Here's how the part is built. I have some questions about the finished solid (model axes, mm). A direction names the side the tool comes from. Coordinates: 2 decimals unless noted, no trailing zeros. Loops run counter-clockwise (first coordinate to the right, second up) from the corner with the lowest first, then second, coordinate; pieces in that order, holes last. Notation, with made-up numbers: M -2.5,-1 L 31.5,-1 A17 cw 31.5,19 Z; hole C 32,33.25 d5. An arc over 180 degrees is marked long. Use CSV: the item, a comma, the result in double quotes. Start each with the question number.
Q1. For pin 1 Ø15 at (x, z) = (669, -549.5) entering from +Y; pin 2 Ø15 at (y, z) = (270.5, -512) entering from -X; pin 3 Ø15 at (x, z) = (668.5, -291) entering from -Y; pin 4 Ø4 at (x, y) = (178, 278.5) entering from +Z, each with a flat end and sliding along its axis, tell me the tip position at first contact or that it passes through.
Q2. If we section it at C-C (x = 64.5): Please give me the cut outline in (y, z), and give its area (3 significant figures).
Q3. If we mould it in two halves opening along X, with no side actions, what happens to faces 1 (the flat face through (-698.5, -267, -389)), 2 (the flat face through (-673, 292.1, -389)), 3 (the flat face through (647.7, 266, -389))? For each: +X half, -X half, draft (parallel to the pull), parting line (faces both ways), or undercut.
Q4. Which directions (+Z, -Z, +X, -X, +Y, -Y) give clear straight access to the entire face, cutting with the end or side of a thin tool? Please do faces 4 (the flat face through (647.7, -267, -389)), 5 (the flat face through (673, 292.1, -389)), 6 (the flat face through (-673, 241.3, -389)).
Q5. If we section it at A-A (z = -466.5): Please give me the cut outline in (x, y).
Q6. Please list where these lines run through material, in increasing order: probe 1 along X at (y, z) = (262.5, -161); probe 2 along Z at (x, y) = (411.5, 45). Write a range as [from, to].
Q7. If we section it at B-B (y = -78): Please give me the cut outline in (x, z), and give its area (3 significant figures).
from build123d import *

# Parameters (mm, degrees)
F0_W     = 1828.8
F0_H     = 762
F1_DEPTH = 25.4
F2_W     = 50.8
F2_H     = 50.8
F3_DEPTH = 762


with BuildPart() as f1:
    # F0 (on Top) → F1 (new body)
    with BuildSketch(Plane.XY):
        Rectangle(F0_W, F0_H)
    extrude(amount=-F1_DEPTH)

    # F2 (on Top) → F3 (join)
    with BuildSketch(Plane.XY):
        with Locations((673.1, 266.7)):
            Rectangle(F2_W, F2_H)
        with Locations((673.1, -266.7)):
            Rectangle(F2_W, F2_H)
        with Locations((-673.1, -266.7)):
            Rectangle(F2_W, F2_H)
        with Locations((-673.1, 266.7)):
            Rectangle(F2_W, F2_H)
    extrude(amount=-F3_DEPTH)


solid = f1.part
Results below:
1,pin 1,"y = 292.1"
1,pin 2,"x = -698.5"
1,pin 3,"y = -292.1"
1,pin 4,"z = 0"
2,outline,"M -381,-25.4 L 381,-25.4 L 381,0 L -381,0 Z"
2,area,"19,400 mm^2"
3,face 1,"-X half"
3,face 2,"draft"
3,face 3,"undercut"
4,face 4,"-Z, +Y, -Y"
4,face 5,"-Z, +X, -X, +Y"
4,face 6,"-Z, +X, -X"
5,outline,"M -698.5,-292.1 L -647.7,-292.1 L -647.7,-241.3 L -698.5,-241.3 Z; M -698.5,241.3 L -647.7,241.3 L -647.7,292.1 L -698.5,292.1 Z; M 647.7,-292.1 L 698.5,-292.1 L 698.5,-241.3 L 647.7,-241.3 Z; M 647.7,241.3 L 698.5,241.3 L 698.5,292.1 L 647.7,292.1 Z"
6,probe 1,"[-698.5, -647.7], [647.7, 698.5]"
6,probe 2,"[-25.4, 0]"
7,outline,"M -914.4,-25.4 L 914.4,-25.4 L 914.4,0 L -914.4,0 Z"
7,area,"46,500 mm^2"
